```python
from build123d import *

# Parameters (mm, degrees)
F0_W     = 89.916
F0_H     = 46.99
F0_W_2   = 24.892
F0_H_2   = 22.098
F1_DEPTH = 1.143
F2_W     = 89.916
F2_H     = 46.99
F2_W_2   = 28.194
F2_H_2   = 22.098
F3_DEPTH = 1.27
F4_R     = 6.35
F5_R     = 1.905
F6_DEPTH = 2.413
F7_R     = 1.27


with BuildPart() as f1:
    # F0 (on Top) → F1 (new body)
    with BuildSketch(Plane.XY):
        with Locations((20.066, 0)):
            Rectangle(F0_W, F0_H)
        Rectangle(F0_W_2, F0_H_2, mode=Mode.SUBTRACT)
        with Locations((40.132, 0)):
            Rectangle(F0_W_2, F0_H_2, mode=Mode.SUBTRACT)
    extrude(amount=F1_DEPTH)

    # F2 (on face) → F3 (join)
    with BuildSketch(Plane.XY.offset(1.143)):
        with Locations((20.066, 0)):
            Rectangle(F2_W, F2_H)
        Rectangle(F2_W_2, F2_H_2, mode=Mode.SUBTRACT)
        with Locations((40.132, 0)):
            Rectangle(F2_W_2, F2_H_2, mode=Mode.SUBTRACT)
    extrude(amount=F3_DEPTH)

    # F4
    f4_edges = [f1.edges().sort_by_distance(p)[0] for p in [
        (-24.892, -23.495, 1.2065),
        (-24.892, 23.495, 1.2065),
        (65.024, -23.495, 1.2065),
        (65.024, 23.495, 1.2065),
    ]]
    fillet(f4_edges, radius=F4_R)

    # F5 (on face) → F6 (cut, through all)
    with BuildSketch(Plane.XY.offset(2.413)):
        with Locations((-18.542, 17.145)):
            Circle(F5_R)
        with Locations((-18.542, -17.145)):
            Circle(F5_R)
        with Locations((58.674, -17.145)):
            Circle(F5_R)
        with Locations((58.674, 17.145)):
            Circle(F5_R)
    extrude(amount=-F6_DEPTH, mode=Mode.SUBTRACT)

    # F7
    f7_edges = [f1.edges().sort_by_distance(p)[0] for p in [
        (-23.032128, 21.635128, 0),
    ]]
    fillet(f7_edges, radius=F7_R)


solid = f1.part
```
The listing builds one solid part. Answer for the finished solid, in the listing's coordinates (mm). A direction names the side the tool comes from. Coordinates: 2 decimals unless noted, no trailing zeros. Write each loop counter-clockwise with the first axis right and the second up, starting at its lowest first coordinate (ties: lowest second). Pieces come first, ordered by that corner, then holes. Notation, with made-up numbers: (67, 19) -> (80, 19) arc R18 ccw to (80, 47) -> close; hole circle Ø6 at (73, 63). An arc over 180 degrees is marked (long way). Write each question's results on one line, items separated by ' | '. Start each with the question number.
1) A tool of negligible diameter and unlimited length cuts with its end or side. For faces 4 (the flat face through (27, 0, 1.143)), 5 (the cylindrical face through (58.261, 15.285, 1.223)), from which of +Z, -Z, +X, -X, +Y, -Y can it reach the whole face along a straight path? Write none if from no direction.
2) Flat-ended cylindrical pins translate along their axes: pin 1 Ø1.8 at (x, y) = (13, 3) entering from +Z; pin 2 Ø4.5 at (x, y) = (58.674, -17.145) entering from +Z; pin 3 Ø1.3 at (y, z) = (1.5, 0.5) entering from +X. Find the tip coordinate at first contact, or state that the pin passes through.
3) A cutting plane is placed at A-A (z = 2). Determine the outline of the cut face in (x, y) (3 decimals).
4) A cutting plane is placed at C-C (y = -4). Determine the outline of the cut face in (x, z) (3 decimals), then the cut area to 3 significant figures.
5) Straight lines are drawn through the part: probe 1 along X at (y, z) = (17, 2); probe 2 along X at (y, z) = (-7.5, 1.35) (3 decimals); probe 3 along Y at (x, z) = (27.5, 2.15) (3 decimals). For each, find the intervals that lie inside material, in ascending order.
6) A cutting plane is placed at B-B (x = 31). Determine the outline of the cut face in (y, z) (3 decimals), then the cut area to 3 significant figures.
7) For a pull along Y with two mould halves and no side action, classify faces 1 (the flat face through (19, 0, 0)), 2 (the cylindrical face through (-23.081, -21.585, 1.85)), 3 (the cylindrical face through (59.7, -15.54, 1.22)) as +Y half, -Y half, draft (parallel to the pull), parting line (faces both ways), or undercut.
Values follow:
1) face 4: +Z | face 5: +Z, -Z
2) pin 1: z = 1.14 | pin 2: z = 2.41 | pin 3: x = 65.02
3) outline: (-24.892, -17.145) arc R6.35 ccw to (-18.542, -23.495) -> (58.674, -23.495) arc R6.35 ccw to (65.024, -17.145) -> (65.024, 17.145) arc R6.35 ccw to (58.674, 23.495) -> (-18.542, 23.495) arc R6.35 ccw to (-24.892, 17.145) -> close; hole circle Ø3.81 at (-18.542, -17.145); hole circle Ø3.81 at (-18.542, 17.145); hole (-14.097, -11.049) -> (14.097, -11.049) -> (14.097, 11.049) -> (-14.097, 11.049) -> close; hole (26.035, -11.049) -> (54.229, -11.049) -> (54.229, 11.049) -> (26.035, 11.049) -> close; hole circle Ø3.81 at (58.674, -17.145); hole circle Ø3.81 at (58.674, 17.145)
4) outline: (-24.892, 1.27) arc R1.27 ccw to (-23.622, 0) -> (-12.446, 0) -> (-12.446, 1.143) -> (-14.097, 1.143) -> (-14.097, 2.413) -> (-24.892, 2.413) -> close; (12.446, 0) -> (27.686, 0) -> (27.686, 1.143) -> (26.035, 1.143) -> (26.035, 2.413) -> (14.097, 2.413) -> (14.097, 1.143) -> (12.446, 1.143) -> close; (52.578, 0) -> (63.754, 0) arc R1.27 ccw to (65.024, 1.27) -> (65.024, 2.413) -> (54.229, 2.413) -> (54.229, 1.143) -> (52.578, 1.143) -> close | area: 87.8 mm²
5) probe 1: -24.89 to -20.44, -16.64 to 56.77, 60.57 to 65.02 | probe 2: -24.892 to -14.097, 14.097 to 26.035, 54.229 to 65.024 | probe 3: -23.495 to -11.049, 11.049 to 23.495
6) outline: (-23.495, 1.27) arc R1.27 ccw to (-22.225, 0) -> (-11.049, 0) -> (-11.049, 2.413) -> (-23.495, 2.413) -> close; (11.049, 0) -> (22.225, 0) arc R1.27 ccw to (23.495, 1.27) -> (23.495, 2.413) -> (11.049, 2.413) -> close | area: 59.4 mm²
7) face 1: draft | face 2: -Y half | face 3: undercut
